Here's how the part is built. I have some questions about the finished solid (model axes, mm). A direction names the side the tool comes from. Coordinates: 2 decimals unless noted, no trailing zeros. Write each loop counter-clockwise with the first axis right and the second up, starting at its lowest first coordinate (ties: lowest second). Pieces come first, ordered by that corner, then holes. Notation, with made-up numbers: (20, 65.25) -> (40, 65.25) arc R23 ccw to (40, 90.25) -> close; hole circle Ø9 at (-12, 21). An arc over 180 degrees is marked (long way). Put each result on its own line as item: value. Start each with the question number.
Item 1: On a 3-axis mill with a long thin cutter (end or side, diameter ignored), from which of +Z, -Z, +X, -X, +Y, -Y can I reach the whole of each face in a straight line? I mean faces 1 (the face through (2550, -1, 30)), 2 (the face through (2509, -1, 0)), 3 (the face through (39, -1, 0)). Say none if no direction works.
Item 2: For pin 1 (1.5 mm diameter, centred on y = 28, z = -15, fed in from +X); pin 2 (4 mm diameter, centred on y = 17.5, z = -17, fed in from -X); pin 3 (24 mm diameter, centred on x = 49, y = -0.5, fed in from -Z), each with a flat end and sliding along its axis, tell me the tip position at first contact or that it passes through.
Item 3: I want a section at A-A, the plane y = 23. List the corners of the cut face in (x, z) for me, then the cut area to 3 significant figures.
Item 4: I need wall thicknesses on line 1 (X direction, y = 22, z = -24.5). Which ranges of the line are inside material? Lowest first, please. Write a range as [from, to].
from build123d import *

# Parameters (mm, degrees)
F0_W     = 80
F0_H     = 120
F1_DEPTH = 2550
F2_W     = 80
F2_H     = 60
F3_DEPTH = 80


with BuildPart() as f1:
    # F0 (on Right) → F1 (new body)
    with BuildSketch(Plane.YZ):
        Rectangle(F0_W, F0_H)
    extrude(amount=F1_DEPTH)

    # F2 (on face) → F3 (cut, through all)
    with BuildSketch(Plane.XZ.offset(40)):
        with Locations((2510, -30)):
            Rectangle(F2_W, F2_H)
        with Locations((40, -30)):
            Rectangle(F2_W, F2_H)
    extrude(amount=-F3_DEPTH, mode=Mode.SUBTRACT)


solid = f1.part
Calculated:
1. face 1: +Z, -Z, +X, +Y, -Y
1. face 2: -Z, +X, +Y, -Y
1. face 3: -Z, -X, +Y, -Y
2. pin 1: stops at x = 2470
2. pin 2: stops at x = 80
2. pin 3: stops at z = 0
3. outline: (0, 0) -> (80, 0) -> (80, -60) -> (2470, -60) -> (2470, 0) -> (2550, 0) -> (2550, 60) -> (0, 60) -> close
3. area: 296,000 mm2
4. line 1: x = [80, 2470]
